CAD build for the part. Positions are in the model's coordinates, mm. A direction names the side the tool comes from. Coordinates: 2 decimals unless noted, no trailing zeros. Loops run counter-clockwise (first coordinate to the right, second up) from the corner with the lowest first, then second, coordinate; pieces in that order, holes last.
1) Saw through at D-D, the plane x = 10.5. Write the cut outline in (y, z), and give its area (3 significant figures).
2) Wall check: line 1 along Z through (x, y) = (39, -27). Give the ranges that are in metal, low to high.
3) Saw through at B-B, the plane x = 31. Write the cut outline in (y, z), and give its area (3 significant figures).
4) Saw through at C-C, the plane z = 27.5. Write the cut outline in (x, y).
5) Saw through at A-A, the plane y = -25. Write the cut outline in (x, z).
6) Which spindle directions (+Z, -Z, +X, -X, +Y, -Y) get a long thin tool onto all of the face, cutting with end or side? Do faces 1 (the cylindrical face through (31.959, -23.803, 28.531)), 2 (the flat face through (16, 8.943, 13)). Say none if no direction does.
7) Two-plate mould, pull along Y, no slides. Class faces 3 (the flat face through (28, -4, 31.75)), 4 (the cylindrical face through (34.6, -1.85, 28.53)), 5 (the flat face through (15, -41.857, 13)): +Y half, -Y half, draft (parallel to the pull), parting line (faces both ways), or undercut.
```python
from build123d import *

# Parameters (mm, degrees)
F0_R     = 6.35
F1_DEPTH = 25.4
F2_DEPTH = 31.75


with BuildPart() as f1:
    # F0 (on Top) → F1 (new body)
    with BuildSketch(Plane.XY):
        Polygon((3.144786, 8.942672), (-9.555214, 8.942672), (-9.555214, -3.757328), (-9.555214, -29.157328), (-9.555214, -41.857328), (3.144786, -41.857328), (28.544786, -41.857328), (41.244786, -41.857328), (41.244786, -29.157328), (41.244786, -3.757328), (41.244786, 8.942672), (28.544786, 8.942672), align=None)
        with Locations((3.144786, -29.157328)):
            Circle(F0_R, mode=Mode.SUBTRACT)
        with Locations((28.544786, -29.157328)):
            Circle(F0_R, mode=Mode.SUBTRACT)
        with Locations((3.144786, -3.757328)):
            Circle(F0_R, mode=Mode.SUBTRACT)
        with Locations((28.544786, -3.757328)):
            Circle(F0_R, mode=Mode.SUBTRACT)
    extrude(amount=F1_DEPTH)

    # F0 (on Top) → F2 (join)
    with BuildSketch(Plane.XY):
        with Locations((28.544786, -29.157328)):
            Circle(F0_R)
        with Locations((3.144786, -3.757328)):
            Circle(F0_R)
        with Locations((28.544786, -3.757328)):
            Circle(F0_R)
        with Locations((3.144786, -29.157328)):
            Circle(F0_R)
    extrude(amount=F2_DEPTH)


solid = f1.part
```
Data:
1. outline: (-41.86, 0) - (8.94, 0) - (8.94, 25.4) - (-41.86, 25.4) - close
1. area: 1,290 mm2
2. line 1: z = 0 to 25.4
3. outline: (-41.86, 0) - (8.94, 0) - (8.94, 25.4) - (2.1, 25.4) - (2.1, 31.75) - (-9.61, 31.75) - (-9.61, 25.4) - (-23.3, 25.4) - (-23.3, 31.75) - (-35.01, 31.75) - (-35.01, 25.4) - (-41.86, 25.4) - close
3. area: 1,440 mm2
4. outline: circle Ø12.7 at (3.14, -29.16); circle Ø12.7 at (3.14, -3.76); circle Ø12.7 at (28.54, -29.16); circle Ø12.7 at (28.54, -3.76)
5. outline: (-9.56, 0) - (41.24, 0) - (41.24, 25.4) - (33.34, 25.4) - (33.34, 31.75) - (23.74, 31.75) - (23.74, 25.4) - (7.94, 25.4) - (7.94, 31.75) - (-1.66, 31.75) - (-1.66, 25.4) - (-9.56, 25.4) - close
6. face 1: +Z
6. face 2: +Z, -Z, +X, -X, +Y
7. face 3: draft
7. face 4: undercut
7. face 5: -Y half
